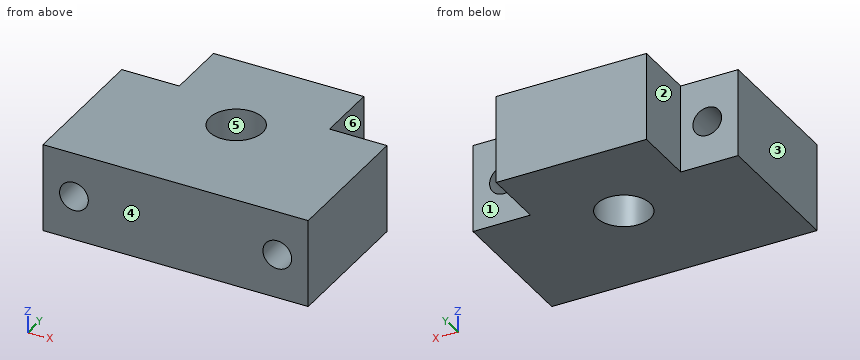
from build123d import *

# Parameters (mm, degrees)
SKETCH_R     = 6
PAD_DEPTH    = 20
SKETCH001_R  = 3.25
POCKET_DEPTH = 32.501


with BuildPart() as part:
    # Sketch → Pad (new body)
    with BuildSketch(Plane.XY):
        Polygon((-17, 21.625642), (17, 21.625642), (17, 7.5), (30, 7.5), (30, -25), (-30, -25), (-30, 7.5), (-17, 7.5), align=None)
        Circle(SKETCH_R, mode=Mode.SUBTRACT)
    extrude(amount=PAD_DEPTH)

    # Sketch001 (on Face7 of Pad) → Pocket (cut, through all)
    with BuildSketch(Plane(origin=(0, 7.5, 0), x_dir=(-1, 0, 0), z_dir=(0, 1, 0))):
        with Locations((-23, 10)):
            Circle(SKETCH001_R)
        with Locations((23, 10)):
            Circle(SKETCH001_R)
    extrude(amount=-POCKET_DEPTH, mode=Mode.SUBTRACT)


solid = part.part
Read the model definition and answer for the solid it produces. Units are mm, in the model's axes. Face numbers are marked on the shaded views. A direction names the side the tool comes from. Give positions to 0.01 mm unless a question says otherwise; leave off trailing zeros. Write each loop counter-clockwise with the first axis right and the second up, starting at its lowest first coordinate (ties: lowest second). Pieces come first, ordered by that corner, then holes. Notation, with made-up numbers: (56, 60) - (111, 60) arc R22 cw to (111, 70) - close; hole circle Ø10 at (40, 67.5). An arc over 180 degrees is marked (long way). Answer in a Markdown table with one row per item. Add a question column.
Item 1: Determine the mould class of the marked faces 4, 5 and 6 for opening direction X: pulls with the +X half, pulls with the -X half, needs draft (parallel to the pull), parting line crosses it, or undercut.
Item 2: Section A-A, the plane z = 10 is taken. Write down the section's boundary in (x, y), and give its area (3 significant figures).
Item 3: Section D-D, the plane z = 3.5 is taken. Write down the section's boundary in (x, y), and give its area (3 significant figures).
Item 4: A tool of negligible diameter and unlimited length cuts with its end or side. For the marked faces 1, 2 and 3, from which of +Z, -Z, +X, -X, +Y, -Y can it reach the whole face along a straight path? Write none if from no direction.
Item 5: Find the intervals of material crossed by L1, parallel to Z at x = -23, y = -14; L2, parallel to Y at x = 0, z = 13; L3, parallel to Y at x = -18, z = 2, in increasing order.
Item 6: Section B-B, the plane y = 0 is taken. Write down the section's boundary in (x, z), and give its area (3 significant figures).
Item 7: Flat-ended cylindrical pins translate along their axes: P1, Ø7, axis at y = 17.5, z = 5, coming from the +X side; P2, Ø12, axis at x = 17.5, z = 5.5, coming from the +Y side; P3, Ø6.5, axis at x = -23.5, z = 10, coming from the +Y side. Find the tip coordinate at first contact, or state that the pin passes through.
Item 8: Section C-C, the plane x = -23 is taken. Write down the section's boundary in (y, z).
Recorded:
| question | item | result |
|---|---|---|
| 1 | face 4 | needs draft |
| 1 | face 5 | undercut |
| 1 | face 6 | pulls with the +X half |
| 2 | outline | (-30, -25) - (-26.25, -25) - (-26.25, 7.5) - (-30, 7.5) - close; (-19.75, -25) - (19.75, -25) - (19.75, 7.5) - (17, 7.5) - (17, 21.63) - (-17, 21.63) - (-17, 7.5) - (-19.75, 7.5) - close; (26.25, -25) - (30, -25) - (30, 7.5) - (26.25, 7.5) - close; hole circle Ø12 at (0, 0) |
| 2 | area | 1,890 mm2 |
| 3 | outline | (-30, -25) - (30, -25) - (30, 7.5) - (17, 7.5) - (17, 21.63) - (-17, 21.63) - (-17, 7.5) - (-30, 7.5) - close; hole circle Ø12 at (0, 0) |
| 3 | area | 2,320 mm2 |
| 4 | face 1 | +Z, -Z, +X, +Y |
| 4 | face 2 | +Z, -Z, -X, +Y |
| 4 | face 3 | +Z, -Z, -X, +Y, -Y |
| 5 | L1 | z = 0 to 6.75, 13.25 to 20 |
| 5 | L2 | y = -25 to -6, 6 to 21.63 |
| 5 | L3 | y = -25 to 7.5 |
| 6 | outline | (-30, 0) - (-6, 0) - (-6, 20) - (-30, 20) - close; (6, 0) - (30, 0) - (30, 20) - (6, 20) - close; hole circle Ø6.5 at (-23, 10); hole circle Ø6.5 at (23, 10) |
| 6 | area | 894 mm2 |
| 7 | P1 | stops at x = 17 |
| 7 | P2 | stops at y = 21.63 |
| 7 | P3 | stops at y = 7.5 |
| 8 | outline | (-25, 0) - (7.5, 0) - (7.5, 6.75) - (-25, 6.75) - close; (-25, 13.25) - (7.5, 13.25) - (7.5, 20) - (-25, 20) - close |
